```python
from build123d import *

# Parameters (mm, degrees)
F0_W     = 277
F0_H     = 5
F1_DEPTH = 5


with BuildPart() as f1:
    # F0 (on Front) → F1 (new body)
    with BuildSketch(Plane.XZ):
        Polygon((-138.5, -279.5), (-138.5, 279.5), (-138.5, 284.5), (-143.5, 284.5), (-143.5, -284.5), (-138.5, -284.5), align=None)
        with Locations((0, 282)):
            Rectangle(F0_W, F0_H)
        Polygon((138.5, 284.5), (138.5, 279.5), (138.5, -279.5), (138.5, -284.5), (143.5, -284.5), (143.5, 284.5), align=None)
        with Locations((0, -282)):
            Rectangle(F0_W, F0_H)
    extrude(amount=F1_DEPTH)


solid = f1.part
```
Here's how the part is built. I have some questions about the finished solid (model axes, mm). Coordinates: 2 decimals unless noted, no trailing zeros. Order: outer loops, then holes, each group sorted by start corner. A loop starts at its lowest first (then second) coordinate and runs counter-clockwise, first axis right, second up. Notation, with made-up numbers: (31.5, 7.5) - (38.5, 7.5) arc R20 cw to (38.5, 15.5) - close; hole circle Ø5 at (34.5, 45.25). An arc over 180 degrees is marked (long way). One line per question, with ' | ' between items.
(1) Suppose I cut it at C-C on x = -89. List the corners of the cut face in (y, z) for me.
Report:
outline: (-5, -284.5) - (0, -284.5) - (0, -279.5) - (-5, -279.5) - close; (-5, 279.5) - (0, 279.5) - (0, 284.5) - (-5, 284.5) - close
(2) If I drill on L1, parallel to Z at x = -12.5, y = -1.8; L2, parallel to X at y = -0.55, z = 143.5, over which ranges is the centre line in solid material (lowest first)?
Report:
L1: z = -284.5 to -279.5, 279.5 to 284.5 | L2: x = -143.5 to -138.5, 138.5 to 143.5
(3) Suppose I cut it at B-B on z = 169.5. List the corners of the cut face in (x, y) for me, and give its area (3 significant figures).
Report:
outline: (-143.5, -5) - (-138.5, -5) - (-138.5, 0) - (-143.5, 0) - close; (138.5, -5) - (143.5, -5) - (143.5, 0) - (138.5, 0) - close | area: 50.0 mm2
(4) Suppose I cut it at A-A on y = -2.8. List the corners of the cut face in (x, z) for me, and give its area (3 significant figures).
Report:
outline: (-143.5, -284.5) - (143.5, -284.5) - (143.5, 284.5) - (-143.5, 284.5) - close; hole (-138.5, -279.5) - (138.5, -279.5) - (138.5, 279.5) - (-138.5, 279.5) - close | area: 8,460 mm2
